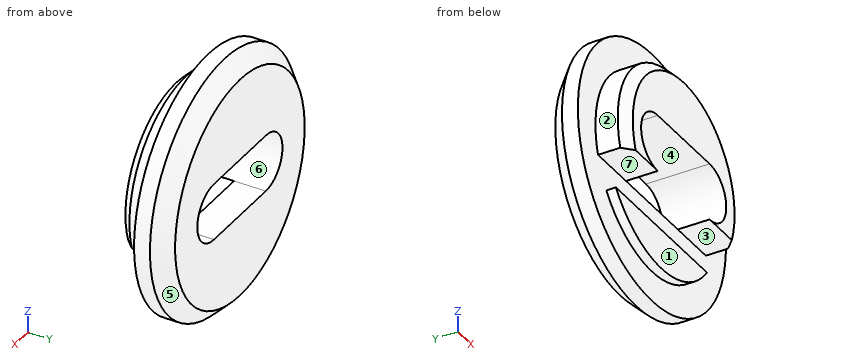
from build123d import *

# Parameters (mm, degrees)
CUT_EXTRUDE1_DEPTH = 13
SKETCH4_W          = 21.205208
SKETCH4_H          = 1.8
CUT_EXTRUDE2_DEPTH = 2
SKETCH5_W          = 20.395214747
SKETCH5_H          = 5.649183718
CUT_EXTRUDE3_DEPTH = 1.4
CHAMFER1_SIZE      = 1
CHAMFER2_SIZE      = 0.6


with BuildPart() as part:
    # Sketch1 → Revolve1 (revolve)
    with BuildSketch(Plane.XY, mode=Mode.PRIVATE) as revolve1_sk:
        Polygon((0, 0), (-8, 0), (-8, -2), (-6.1, -2), (-6.1, -4), (0, -4), align=None)
    revolve(revolve1_sk.sketch.rotate(Axis((0, 0, 0), (0, -1, 0)), 270), axis=Axis((0, 0, 0), (0, -1, 0)))

    # Sketch3 → Cut-Extrude1 (cut, through all)
    with BuildSketch(Plane(origin=(0, 0, 0), x_dir=(1, 0, 0), z_dir=(0, 1, 0))):
        with BuildLine():
            Line((-2.8, 1.8), (2.8, 1.8))
            ThreePointArc((2.8, 1.8), (4.6, 0), (2.8, -1.8))
            Line((2.8, -1.8), (-2.8, -1.8))
            ThreePointArc((-2.8, -1.8), (-4.6, 0), (-2.8, 1.8))
        make_face()
    extrude(amount=-CUT_EXTRUDE1_DEPTH, mode=Mode.SUBTRACT)

    # Sketch4 → Cut-Extrude2 (cut)
    with BuildSketch(Plane.XZ.offset(4)):
        with Locations((0.56076456, -2.7)):
            Rectangle(SKETCH4_W, SKETCH4_H)
    extrude(amount=-CUT_EXTRUDE2_DEPTH, mode=Mode.SUBTRACT)

    # Sketch5 → Cut-Extrude3 (cut)
    with BuildSketch(Plane.XZ.offset(4)):
        with Locations((-0.031153587, -4.97418934)):
            Rectangle(SKETCH5_W, SKETCH5_H)
    extrude(amount=-CUT_EXTRUDE3_DEPTH, mode=Mode.SUBTRACT)

    # Chamfer1
    chamfer1_edges = [part.edges().sort_by_distance(p)[0] for p in [
        (0, 0, -8),
    ]]
    chamfer(chamfer1_edges, length=CHAMFER1_SIZE)

    # Chamfer2
    chamfer2_edges = [part.edges().sort_by_distance(p)[0] for p in [
        (0, -4, 6.1),
    ]]
    chamfer(chamfer2_edges, length=CHAMFER2_SIZE)


solid = part.part
Could you check a few things on this model? Use its own coordinates, in mm. Face numbers are marked on the shaded views. A direction names the side the tool comes from. Round coordinates to 2 decimals unless told otherwise and drop trailing zeros. Order: outer loops, then holes, each group sorted by start corner. A loop starts at its lowest first (then second) coordinate and runs counter-clockwise, first axis right, second up. Notation, with made-up numbers: M -27,32 L 28,32 A9 cw 28,42 Z; hole C 6.5,1.25 d11. An arc over 180 degrees is marked long. One line per item, written item: value.
(1) I'm going to push flat-ended pins straight in: P1, Ø5, axis at x = -3.5, z = -3.5, coming from the +Y side; P2, Ø1.5, axis at x = -1.5, y = -3, coming from the +Z side; P3, Ø0.6, axis at x = 5, y = -3.5, coming from the -Z side; P4, Ø2, axis at x = 1, z = -4.5, coming from the -Y side. Where does each tip first touch, or does it pass through?
Ans:
P1: stops at y = 0
P2: stops at z = 6.05
P3: stops at z = -1.8
P4: stops at y = -2.6
(2) Imagine slicing it at C-C (y = -3.6). Write out the boundary of the cut face in (x, z), and give its area (3 significant figures).
Ans:
outline: M -5.62,-1.8 L -2.8,-1.8 A1.8 cw -2.8,1.8 L 2.8,1.8 A1.8 cw 2.8,-1.8 L 5.62,-1.8 A5.9 ccw long Z
area: 45.2 mm^2
(3) If we mould it in two halves opening along X, with no side actions, what happens to the marked faces 5, 6 and 7? For each: released by +X, released by -X, zero draft, split by the parting line, or undercut.
Ans:
face 5: split by the parting line
face 6: undercut
face 7: zero draft
(4) Imagine slicing it at A-A (z = 0). Write out the boundary of the cut face in (x, y), and give its area (3 significant figures).
Ans:
outline: M -8,-2 L -6.1,-2 L -6.1,-3.4 L -5.5,-4 L -4.6,-4 L -4.6,0 L -7,0 L -8,-1 Z; M 4.6,-4 L 5.5,-4 L 6.1,-3.4 L 6.1,-2 L 8,-2 L 8,-1 L 7,0 L 4.6,0 Z
area: 18.2 mm^2
(5) Imagine slicing it at B-B (y = -0.55). Write out the boundary of the cut face in (x, z).
Ans:
outline: C 0,0 d15.1; hole M -2.8,-1.8 L 2.8,-1.8 A1.8 ccw 2.8,1.8 L -2.8,1.8 A1.8 ccw Z
(6) Which directions (+Z, -Z, +X, -X, +Y, -Y) give clear straight access to the entire face, cutting with the end or side of a thin tool? Please do the marked faces 1, 2, 3 and 4.
Ans:
face 1: -Z, +X, -X, -Y
face 2: -Y
face 3: +X, -X, -Y
face 4: +Y, -Y
(7) I need wall thicknesses on line 1 along X through (y, z) = (-3.2, 0); line 2 along Y through (x, z) = (4.25, -4.5); line 3 along Y through (x, z) = (-0.25, -5.5). Which ranges of each line are inside material? Lowest first, please. Write a range as from..to.
Ans:
line 1: x = -6.1..-4.6, 4.6..6.1
line 2: y = -2..0
line 3: y = -2.6..0
